Read the model definition and answer for the solid it produces. Units are mm, in the model's axes. Coordinates: 2 decimals unless noted, no trailing zeros. Loops run counter-clockwise (first coordinate to the right, second up) from the corner with the lowest first, then second, coordinate; pieces in that order, holes last. Notation, with made-up numbers: (69.5, 11.5) - (118.5, 11.5) arc R17 cw to (118.5, 38.5) - close; hole circle Ø6 at (-17, 75.5). An arc over 180 degrees is marked (long way). Use CSV: the item, a comma, the result in double quotes.
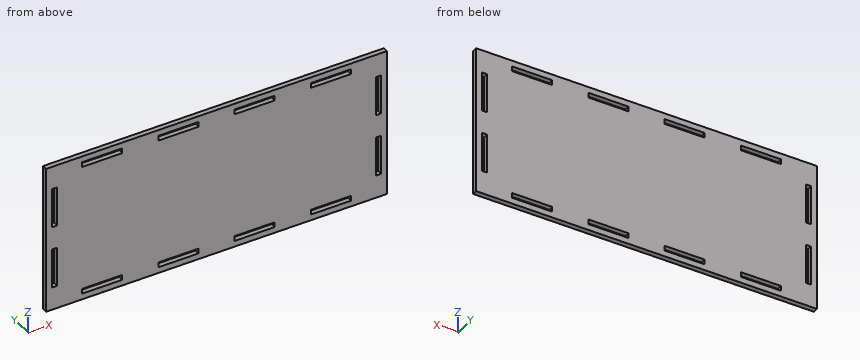
```python
from build123d import *

# Parameters (mm, degrees)
F0_W     = 215.9
F0_H     = 95.25
F0_W_2   = 25.4254
F0_H_2   = 3.2004
F0_W_3   = 3.2004
F0_H_3   = 25.4254
F1_DEPTH = 3.175


with BuildPart() as f1:
    # F0 (on Front) → F1 (new body)
    with BuildSketch(Plane.XZ):
        with Locations((10.806967, -3.292766)):
            Rectangle(F0_W, F0_H)
        with Locations((-61.590653, -45.507566)):
            Rectangle(F0_W_2, F0_H_2, mode=Mode.SUBTRACT)
        with Locations((-13.325573, -45.507566)):
            Rectangle(F0_W_2, F0_H_2, mode=Mode.SUBTRACT)
        with Locations((-91.732833, -23.407026)):
            Rectangle(F0_W_3, F0_H_3, mode=Mode.SUBTRACT)
        with Locations((34.939507, -45.507566)):
            Rectangle(F0_W_2, F0_H_2, mode=Mode.SUBTRACT)
        with Locations((83.204587, -45.507566)):
            Rectangle(F0_W_2, F0_H_2, mode=Mode.SUBTRACT)
        with Locations((113.346767, -23.407026)):
            Rectangle(F0_W_3, F0_H_3, mode=Mode.SUBTRACT)
        with Locations((-91.732833, 16.818954)):
            Rectangle(F0_W_3, F0_H_3, mode=Mode.SUBTRACT)
        with Locations((-61.590653, 38.922034)):
            Rectangle(F0_W_2, F0_H_2, mode=Mode.SUBTRACT)
        with Locations((-13.325573, 38.922034)):
            Rectangle(F0_W_2, F0_H_2, mode=Mode.SUBTRACT)
        with Locations((113.346767, 16.818954)):
            Rectangle(F0_W_3, F0_H_3, mode=Mode.SUBTRACT)
        with Locations((34.939507, 38.922034)):
            Rectangle(F0_W_2, F0_H_2, mode=Mode.SUBTRACT)
        with Locations((83.204587, 38.922034)):
            Rectangle(F0_W_2, F0_H_2, mode=Mode.SUBTRACT)
    extrude(amount=F1_DEPTH)


solid = f1.part
```
Q1. Find the intervals of material crossed by probe 1 along Z at (x, y) = (83, -0.3); probe 2 along X at (y, z) = (-0.8, -17), in increasing order. Write a range as [from, to].
Reported:
probe 1,"z = [-50.92, -47.11], [-43.91, 37.32], [40.52, 44.33]"
probe 2,"x = [-97.14, -93.33], [-90.13, 111.75], [114.95, 118.76]"
Q2. The part is cut by section A-A on z = -20.5. Determine the outline of the cut face in (x, y) (3 decimals).
Reported:
outline,"(-97.143, -3.175) - (-93.333, -3.175) - (-93.333, 0) - (-97.143, 0) - close; (-90.133, -3.175) - (111.747, -3.175) - (111.747, 0) - (-90.133, 0) - close; (114.947, -3.175) - (118.757, -3.175) - (118.757, 0) - (114.947, 0) - close"
Q3. The part is cut by section B-B on x = 30. Determine the outline of the cut face in (y, z) (3 decimals), and give its area (3 significant figures).
Reported:
outline,"(-3.175, -50.918) - (0, -50.918) - (0, -47.108) - (-3.175, -47.108) - close; (-3.175, -43.907) - (0, -43.907) - (0, 37.322) - (-3.175, 37.322) - close; (-3.175, 40.522) - (0, 40.522) - (0, 44.332) - (-3.175, 44.332) - close"
area,"282 mm²"
Q4. The part is cut by section C-C on y = -2. Give the number of separate pieces and of enclosed holes in the cut face, and give its area (3 significant figures).
Reported:
separate pieces,"1"
enclosed holes,"12"
area,"19,600 mm²"
